Can you work these out from the model? Positions are in its coordinate system, mm. Face numbers are marked on the shaded views. A direction names the side the tool comes from. Coordinates: 2 decimals unless noted, no trailing zeros. Order: outer loops, then holes, each group sorted by start corner. A loop starts at its lowest first (then second) coordinate and runs counter-clockwise, first axis right, second up. Notation, with made-up numbers: (-18, -26) -> (19, -26) arc R8 cw to (19, -16) -> close; hole circle Ø6 at (85.25, 38). An arc over 180 degrees is marked (long way). Answer in a Markdown table with one row per item. Add a question column.
1. Imagine slicing it at A-A on z = -17. Write out the boundary of the cut face in (x, y), plus the area to 3 significant figures.
2. Imagine slicing it at D-D on x = -10.5. Write out the boundary of the cut face in (y, z), plus the area to 3 significant figures.
3. Imagine slicing it at B-B on x = 7.5. Write out the boundary of the cut face in (y, z).
4. Imagine slicing it at C-C on y = -1.5. Write out the boundary of the cut face in (x, z), plus the area to 3 significant figures.
5. Will these pins go through, and if not, where does the flat tip stop? pin 1 (2.5 mm diameter, centred on y = -9, z = -17, fed in from +X); pin 2 (6.5 mm diameter, centred on y = -9.5, z = -16, fed in from -X); pin 3 (5 mm diameter, centred on y = -8, z = 17, fed in from +X); pin 4 (4.5 mm diameter, centred on x = -10, z = 10, fed in from -Y).
6. On a 3-axis mill with a long thin cutter (end or side, diameter ignored), from which of +Z, -Z, +X, -X, +Y, -Y can I reach the whole of each face in a straight line? I mean the marked faces 4 and 5. Say none if no direction works.
7. We'd pull the mould along Z, two halves only. Please class the marked faces 1, 2 and 3: pulls with the +Z half, pulls with the -Z half, needs draft (parallel to the pull), parting line crosses it, or undercut.
8. If I drill on line 1 along Z through (x, y) = (-10, -3.45); line 2 along Z through (x, y) = (-1.75, -9); line 3 along Z through (x, y) = (9.5, -8), over which ranges is the centre line in solid material (lowest first)? Write a range as [from, to].
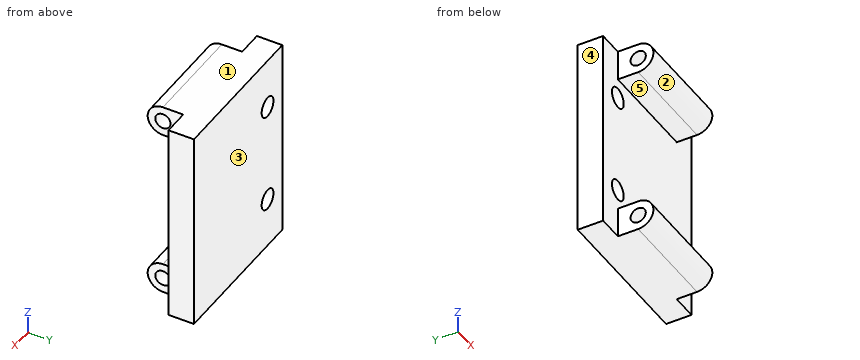
from build123d import *

# Parameters (mm, degrees)
SKETCH_W          = 30
SKETCH_H          = 40
PAD_DEPTH         = 5
PAD001_DEPTH      = 10
SKETCH002_R       = 1.5
POCKET_DEPTH      = 117.840681
POCKET_DEPTH_BACK = 117.840681
SKETCH003_R       = 2
POCKET001_DEPTH   = 12.001


with BuildPart() as part:
    # Sketch (on DatumPlane) → Pad (new body)
    with BuildSketch(Plane.XZ):
        Rectangle(SKETCH_W, SKETCH_H)
    extrude(amount=PAD_DEPTH)

    # Sketch001 (on DatumPlane) → Pad001 (join, symmetric)
    with BuildSketch(Plane.YZ):
        with BuildLine():
            Line((-9, 20), (-5, 20))
            Line((-5, 20), (-5, 14))
            Line((-5, 14), (-9, 14))
            ThreePointArc((-9, 20), (-12, 17), (-9, 14))
        make_face()
    pad001 = extrude(amount=PAD001_DEPTH, both=True)

    # Sketch002 (on DatumPlane) → Pocket (cut, two sides)
    with BuildSketch(Plane.YZ) as pocket_sk:
        with Locations((-9, 17)):
            Circle(SKETCH002_R)
    pocket = extrude(amount=-POCKET_DEPTH, mode=Mode.SUBTRACT) + extrude(pocket_sk.sketch, amount=POCKET_DEPTH_BACK, mode=Mode.SUBTRACT)

    # Mirrored: Pad001, Pocket across XY
    add(pad001.mirror(Plane.XY))
    add(pocket.mirror(Plane.XY), mode=Mode.SUBTRACT)

    # Sketch003 (on DatumPlane) → Pocket001 (cut, through all)
    with BuildSketch(Plane.XZ):
        with Locations((-10, 10)):
            Circle(SKETCH003_R)
        with Locations((-10, -10)):
            Circle(SKETCH003_R)
    extrude(amount=POCKET001_DEPTH, mode=Mode.SUBTRACT)


solid = part.part
Answers follow:
| question | item | result |
|---|---|---|
| 1 | outline | (-15, -5) -> (-10, -5) -> (-10, -7.5) -> (10, -7.5) -> (10, -5) -> (15, -5) -> (15, 0) -> (-15, 0) -> close; (-10, -12) -> (10, -12) -> (10, -10.5) -> (-10, -10.5) -> close |
| 1 | area | 230 mm² |
| 2 | outline | (-5, -20) -> (0, -20) -> (0, -11.94) -> (-5, -11.94) -> close; (-5, -8.06) -> (0, -8.06) -> (0, 8.06) -> (-5, 8.06) -> close; (-5, 11.94) -> (0, 11.94) -> (0, 20) -> (-5, 20) -> close |
| 2 | area | 161 mm² |
| 3 | outline | (-9, -20) -> (0, -20) -> (0, 20) -> (-9, 20) arc R3 ccw to (-9, 14) -> (-5, 14) -> (-5, -14) -> (-9, -14) arc R3 ccw to start; hole circle Ø3 at (-9, -17); hole circle Ø3 at (-9, 17) |
| 4 | outline | (-15, -20) -> (15, -20) -> (15, 20) -> (-15, 20) -> close; hole circle Ø4 at (-10, -10); hole circle Ø4 at (-10, 10) |
| 4 | area | 1,170 mm² |
| 5 | pin 1 | passes through |
| 5 | pin 2 | stops at x = -10 |
| 5 | pin 3 | stops at x = 10 |
| 5 | pin 4 | stops at y = -5 |
| 6 | face 4 | +Z, -Z, -X, +Y, -Y |
| 6 | face 5 | +X, -X, -Y |
| 7 | face 1 | pulls with the +Z half |
| 7 | face 2 | undercut |
| 7 | face 3 | needs draft |
| 8 | line 1 | z = [-20, -12], [-8, 8], [12, 20] |
| 8 | line 2 | z = [-20, -18.5], [-15.5, -14], [14, 15.5], [18.5, 20] |
| 8 | line 3 | z = [-20, -18.12], [-15.88, -14], [14, 15.88], [18.12, 20] |
